Job drawing, mm, ordinate dimensions from the low corner. One solid piece. Give positions to 0.01 mm unless a question says otherwise; leave off trailing zeros. Order: outer loops, then holes, each group sorted by start corner. A loop starts at its lowest first (then second) coordinate and runs counter-clockwise, first axis right, second up.
Item 1: Flat gauge pins, fed straight in: P1, Ø1, axis at y = 9.5, z = 7, coming from the -X side; P2, Ø6, axis at y = 15.5, z = 11, coming from the +X side; P3, Ø6, axis at y = 36.5, z = 10.5, coming from the -X side. Where does each tip first touch, or does it go through?
Item 2: Band-saw the part on A-A on z = 5. Give the cut face in (x, y).
Item 3: Wall check: L1, parallel to X at y = 58.5, z = 10; L2, parallel to X at y = 18.5, z = 5.5; L3, parallel to Z at x = 16, y = 26. Give the ranges that are in metal, low to high.
Item 4: Band-saw the part on C-C on y = 36. Give the cut face in (x, z).
Item 5: Two-plate mould, pull along X, no slides. Class the marked faces 1, 2 and 3: released by +X, released by -X, zero draft, split by the parting line, or undercut.
Item 6: Band-saw the part on B-B on x = 16. Give the cut face in (y, z).
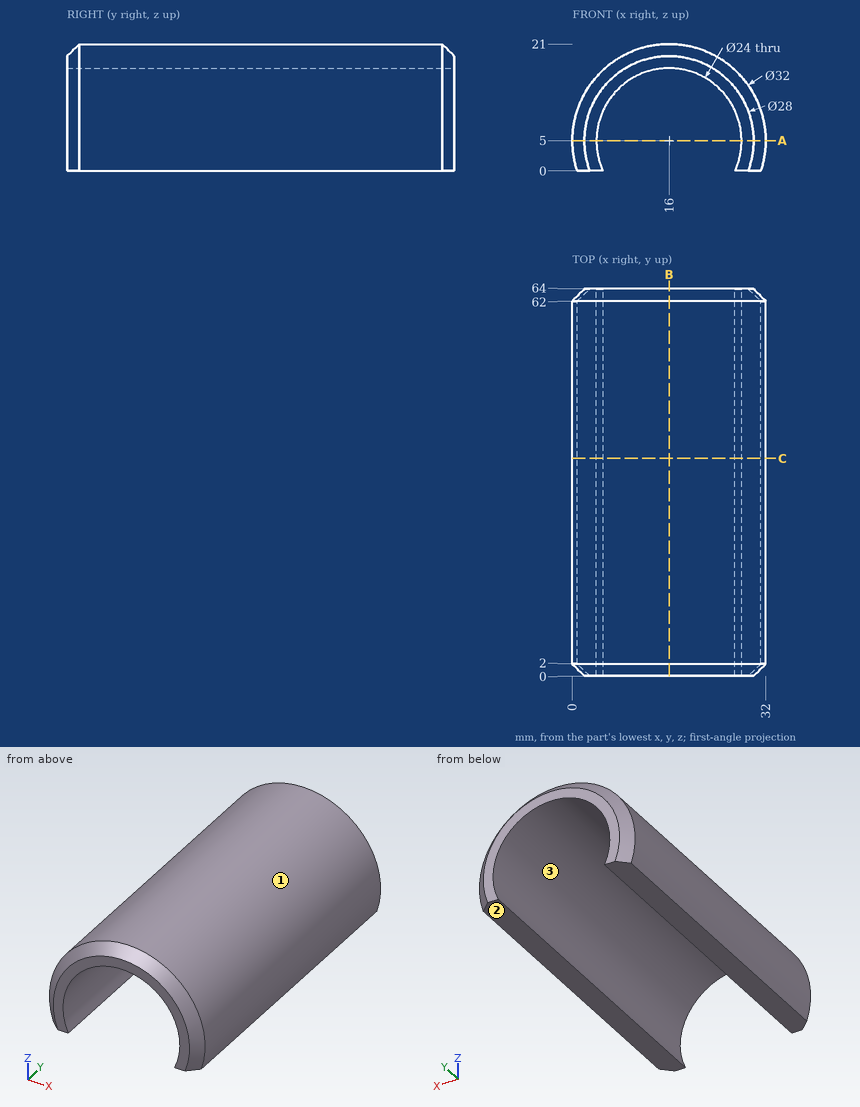
The answers:
1. P1: stops at x = 0.07
1. P2: stops at x = 31.72
1. P3: stops at x = 0.2
2. outline: (0, 2) - (2, 0) - (4, 0) - (4, 64) - (2, 64) - (0, 62) - close; (28, 0) - (30, 0) - (32, 2) - (32, 62) - (30, 64) - (28, 64) - close
3. L1: x = 0.8 to 5.09, 26.91 to 31.2
3. L2: x = 0.01 to 4.01, 27.99 to 31.99
3. L3: z = 17 to 21
4. outline: (0.8, 0) - (5.09, 0) arc R12 cw (long way) to (26.91, 0) - (31.2, 0) arc R16 ccw (long way) to start
5. face 1: split by the parting line
5. face 2: zero draft
5. face 3: undercut
6. outline: (0, 17) - (64, 17) - (64, 19) - (62, 21) - (2, 21) - (0, 19) - close
